```python
from build123d import *

# Parameters (mm, degrees)
F1_DEPTH = 25.4
F2_T     = -1.5875
F3_W     = 22.225
F3_H     = 22.225
F4_DEPTH = 262.563512
F6_DEPTH = 25.4


with BuildPart() as f1:
    # F0 (on Top) → F1 (new body)
    with BuildSketch(Plane.XY):
        Polygon((5.260512, 127.561512), (-12.7, 109.601), (-12.7, -135.001), (12.7, -135.001), (12.7, 120.122024), align=None)
    extrude(amount=F1_DEPTH)

    # F2
    f2_openings = [f1.faces().sort_by_distance(p)[0] for p in [
        (0, -135.001, 12.7),
    ]]
    offset(amount=F2_T, openings=f2_openings)

    # F3 (on face) → F4 (cut, through all)
    with BuildSketch(Plane.XZ.offset(135.001)):
        with Locations((0, 12.7)):
            Rectangle(F3_W, F3_H)
    extrude(amount=-F4_DEPTH, mode=Mode.SUBTRACT)

    # F5 (on face) → F6 (cut)
    with BuildSketch(Plane.XY.offset(25.4)):
        Polygon((5.260512, -117.040488), (-12.7, -135.001), (12.7, -135.001), (12.7, -109.601), align=None)
        Polygon((-12.7, -99.079976), (-12.7, -135.001), (5.260512, -117.040488), align=None)
    extrude(amount=-F6_DEPTH, mode=Mode.SUBTRACT)


solid = f1.part
```
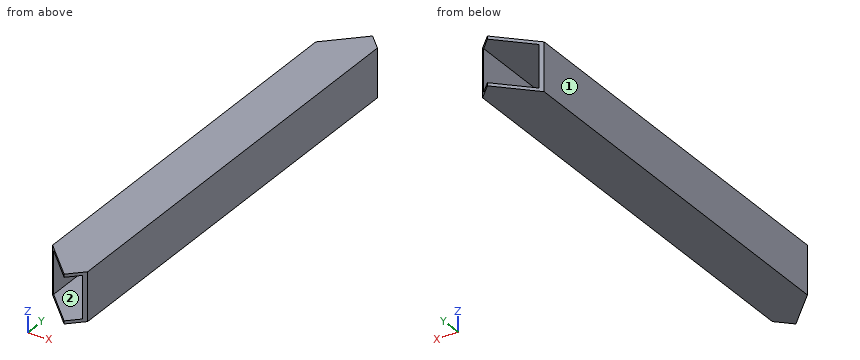
Work out the finished part from the listing and answer in its coordinate system (mm). Face numbers are marked on the shaded views. A direction names the side the tool comes from. Coordinates: 2 decimals unless noted, no trailing zeros. Loops run counter-clockwise (first coordinate to the right, second up) from the corner with the lowest first, then second, coordinate; pieces in that order, holes last. Notation, with made-up numbers: M 66.25,38 L 116.25,38 A32 ccw 116.25,67 Z; hole C 43.5,23.25 d7. An arc over 180 degrees is marked long. Use CSV: the item, a comma, the result in double quotes. Start each with the question number.
(1) Find section B-B, the plane x = 2.75. Give the vertices of the cut face in (y, z), then the cut area to 3 significant figures.
(2) Given pin 1 Ø5 at (x, z) = (-1, 3.5) entering from -Y; pin 2 Ø12 at (x, z) = (-5, 3.5) entering from +Y; pin 3 Ø4 at (x, z) = (-3, 2.5) entering from +Y, each flat-ended and moving along its own axis, determine where each tip first touches the part or whether it passes through.
(3) Find section A-A, the plane z = 8. Give the vertices of the cut face in (x, y).
(4) Find section C-C, the plane y = -18.5. Give the vertices of the cut face in (x, z).
(5) Consider line 1 (X direction, y = -38.5, z = 6); line 2 (Z direction, x = 8.5, y = 3); line 3 (X direction, y = -105, z = 18.75). Determine where each line is inside the solid, lowest interval first.
(6) For the marked faces 1 and 2, determine the directions among +Z, -Z, +X, -X, +Y, -Y from which every point of the face is accessible in a straight line to the end or side of a thin tool.
Recorded:
1,outline,"M -114.53,0 L 125.05,0 L 125.05,1.59 L -114.53,1.59 Z; M -114.53,23.81 L 125.05,23.81 L 125.05,25.4 L -114.53,25.4 Z"
1,area,"761 mm^2"
2,pin 1,"stops at y = -112.39"
2,pin 2,"stops at y = 122.99"
2,pin 3,"stops at y = 121.08"
3,outline,"M -12.7,-99.08 L -11.11,-100.67 L -11.11,111.19 L -12.7,109.6 Z; M 11.11,-111.19 L 12.7,-109.6 L 12.7,120.12 L 11.11,121.71 Z"
4,outline,"M -12.7,0 L 12.7,0 L 12.7,25.4 L -12.7,25.4 Z; hole M -11.11,1.59 L 11.11,1.59 L 11.11,23.81 L -11.11,23.81 Z"
5,line 1,"x = -12.7 to -11.11, 11.11 to 12.7"
5,line 2,"z = 0 to 1.59, 23.81 to 25.4"
5,line 3,"x = 11.11 to 12.7"
6,face 1,"+Z, -Z, -X, +Y, -Y"
6,face 2,"+Y, -Y"
